The model under review builds one solid part; all positions refer to its coordinate system, in mm. A direction names the side the tool comes from. Round coordinates to 2 decimals unless told otherwise and drop trailing zeros. Return JSON: item names as keys, results as strings. Group by question number.
1. Mouldability with a two-part tool opening along Z and no side actions: class faces 1 (the flat face through (72.929, -7, -4)), 2 (the flat face through (-6.157, 5, 2)) as pulls with the +Z half, pulls with the -Z half, needs draft (parallel to the pull), parting line crosses it, or undercut.
2. Tool access review of faces 3 (the flat face through (72.929, 8, 0)), 4 (the flat face through (83.705, 0, 0)): name each direction out of +Z, -Z, +X, -X, +Y, -Y from which nothing blocks a thin tool from reaching the whole face with its end or side.
3. For line 1 along Y through (x, z) = (60, 0); line 2 along Z through (x, y) = (8, 0); line 3 along Y through (x, z) = (66.5, 5.75), list the stretches that pass through material, from the lowest coordinate up. Write a range as from..to.
4. Clearance check with flat-ended pins moving along their axes: P1, Ø1.5, axis at x = 7.5, z = -6, coming from the +Y side; P2, Ø2, axis at x = 48.5, z = -1, coming from the -Y side; P3, Ø2, axis at x = 32, y = -5, coming from the +Z side. State where each tip first meets the part, or that it passes through.
from build123d import *

# Parameters (mm, degrees)
BASPROSKE_W         = 59.315
BASPROSKE_H         = 7
TOOTHCUT_DEPTH      = 61.135424044
TEETHCUTS_COUNT     = 12
TEETHCUTS_ANGLE     = 330
BORSKE_R            = 0.4
BORE_DEPTH          = 50.0000508
SCALE1_SCALE        = 2
BOSS_EXTRUDE1_START = 16.163
SKETCH9_R           = 14
BOSS_EXTRUDE1_DEPTH = 16.163
SCALE2_SCALE        = 0.666666667
SKETCH10_R          = 5
CUT_EXTRUDE1_DEPTH  = 4
CUT_EXTRUDE3_DEPTH  = 20.25


with BuildPart() as part:
    # BasProSke → Base-Revolve (revolve)
    with BuildSketch(Plane(origin=(0, 0, 0), x_dir=(1, 0, 0), z_dir=(0, 1, 0)), mode=Mode.PRIVATE) as base_revolve_sk:
        with Locations((29.6575, 3.5)):
            Rectangle(BASPROSKE_W, BASPROSKE_H)
    revolve(base_revolve_sk.sketch.rotate(Axis((-10, 0, 0), (1, 0, 0)), 180), axis=Axis((-10, 0, 0), (1, 0, 0)))

    # TooCutSke → ToothCut (cut, through all)
    with BuildSketch(Plane(origin=(0, 0, 0), x_dir=(0, 0, -1), z_dir=(1, 0, 0))):
        with BuildLine():
            ThreePointArc((0.562207301, 4.715604304), (0, 4.749), (-0.562207301, 4.715604304))
            ThreePointArc((-0.562207301, 4.715604304), (-0.837528627, 5.917009812), (-1.672850686, 6.823328788))
            ThreePointArc((-1.672850686, 6.823328788), (0, 7.0254), (1.672850686, 6.823328788))
            ThreePointArc((1.672850686, 6.823328788), (0.837528627, 5.917009812), (0.562207301, 4.715604304))
        make_face()
    toothcut = extrude(amount=TOOTHCUT_DEPTH, mode=Mode.SUBTRACT)

    # TeethCuts: ToothCut ×12 about axis
    teethcuts_axis = Axis((-10, 0, 0), (1, 0, 0))
    for i in range(1, TEETHCUTS_COUNT):
        add(toothcut.rotate(teethcuts_axis, i * TEETHCUTS_ANGLE / (TEETHCUTS_COUNT - 1)), mode=Mode.SUBTRACT)

    # BorSke → Bore (cut, symmetric)
    with BuildSketch(Plane(origin=(0, 0, 0), x_dir=(0, 0, -1), z_dir=(1, 0, 0))):
        Circle(BORSKE_R)
    extrude(amount=BORE_DEPTH, both=True, mode=Mode.SUBTRACT)


with BuildPart() as part_1:
    # Scale1: scaled about (29.676274456, 0, 0)
    add(part.part.scale(SCALE1_SCALE).moved(Location((-29.676274456, 0, 0))))

    # Sketch9 → Boss-Extrude1 (add)
    with BuildSketch(Plane(origin=(88.953725544, 0, 0), x_dir=(0, 0, -1), z_dir=(1, 0, 0)).offset(BOSS_EXTRUDE1_START)):
        with Locations(Location((0, 0, 0), (0, 0, 166.421298953))):
            Circle(SKETCH9_R)
    extrude(amount=-BOSS_EXTRUDE1_DEPTH)


with BuildPart() as part_2:
    # Scale2: scaled about (40.880908015, 0, 0)
    add(part_1.part.scale(SCALE2_SCALE).moved(Location((13.626969338, 0, 0))))

    # Sketch10 → Cut-Extrude1 (cut)
    with BuildSketch(Plane.ZY.offset(6.157213633)):
        Circle(SKETCH10_R)
    extrude(amount=-CUT_EXTRUDE1_DEPTH, mode=Mode.SUBTRACT)

    # Sketch11 → Cut-Extrude3 (cut)
    with BuildSketch(Plane.ZY.offset(2.157213633)):
        with BuildLine():
            Line((4.5, 0), (4.5, 2.179449472))
            ThreePointArc((4.5, 2.179449472), (-5, 0), (4.5, -2.179449472))
            Line((4.5, -2.179449472), (4.5, 0))
        make_face()
    extrude(amount=-CUT_EXTRUDE3_DEPTH, mode=Mode.SUBTRACT)


solid = part_2.part
Output:
{
 "1": {"face 1": "undercut", "face 2": "needs draft"},
 "2": {"face 3": "-X, +Y", "face 4": "+Z, -Z, +X, +Y, -Y"},
 "3": {"line 1": "y = -6.33..-0.53, 0.53..6.33", "line 2": "z = -6.33..-5, 4.5..6.33", "line 3": "y = -6.65..-4.28, -2.65..2.65, 4.28..6.65"},
 "4": {"P1": "stops at y = 6.76", "P2": "stops at y = -8.94", "P3": "stops at z = 6.71"}
}
